```python
from build123d import *

# Parameters (mm, degrees)
SKETCH2_R               = 15
CUT_EXTRUDE1_DEPTH      = 10
CUT_EXTRUDE2_DEPTH      = 5.55
CUT_EXTRUDE2_DEPTH_BACK = 5.55


with BuildPart() as part:
    # Sketch1 → Revolve1 (revolve)
    with BuildSketch(Plane.XY, mode=Mode.PRIVATE) as revolve1_sk:
        Polygon((0, 0), (-50, 0), (-50, 30), (0, 15), align=None)
    revolve(revolve1_sk.sketch.rotate(Axis((0, 0, 0), (-1, 0, 0)), 90), axis=Axis((0, 0, 0), (-1, 0, 0)))

    # Sketch2 → Cut-Extrude1 (cut)
    with BuildSketch(Plane.ZY.offset(50)):
        Circle(SKETCH2_R)
    extrude(amount=-CUT_EXTRUDE1_DEPTH, mode=Mode.SUBTRACT)

    # Sketch4 → Cut-Extrude2 (cut, two sides: drawn at the far end of the back side and taken through both)
    with BuildSketch(Plane.XY.offset(-CUT_EXTRUDE2_DEPTH_BACK)):
        Polygon((0, 15), (0, 12), (-50, 27), (-50, 30), align=None)
        Polygon((0, -15), (0, -12), (-50, -27), (-50, -30), align=None)
    extrude(amount=CUT_EXTRUDE2_DEPTH + CUT_EXTRUDE2_DEPTH_BACK, mode=Mode.SUBTRACT)


solid = part.part
```
Could you check a few things on this model? Use its own coordinates, in mm. A direction names the side the tool comes from. Give positions to 0.01 mm unless a question says otherwise; leave off trailing zeros. Order: outer loops, then holes, each group sorted by start corner. A loop starts at its lowest first (then second) coordinate and runs counter-clockwise, first axis right, second up.
Q1. For faces 1 (the flat face through (-25, 21, 5.55)), 2 (the flat face through (-24.65, -19.395, -0.078)), 3 (the cylindrical face through (-45.07, 0.66, -14.985)), which set-ups out of +Z, -Z, +X, -X, +Y, -Y let a thin tool reach every point of the face, with its end or its side?
Q2. We'd pull the mould along Y, two halves only. Please class faces 4 (the flat face through (-25, 21, -5.55)), 5 (the flat face through (-40, 0, 0)), 6 (the conical face through (-24.65, -0.43, 22.39)): +Y half, -Y half, draft (parallel to the pull), parting line (faces both ways), or undercut.
Q3. Suppose I cut it at A-A, the plane y = 0. Write out the boundary of the cut face in (x, z).
Q4. Suppose I cut it at B-B, the plane z = 0. Write out the boundary of the cut face in (x, y).
Q5. I'm going to push flat-ended pins straight in: P1, Ø2, axis at x = -17.5, z = -6.5, coming from the +Y side; P2, Ø3, axis at x = -23, y = -20, coming from the +Z side; P3, Ø5, axis at x = -34.5, y = 23, coming from the -Z side; P4, Ø5, axis at x = -17, y = -22.5, coming from the +Z side. Where does each tip first touch, or does it pass through?
Q6. If I drill on line 1 along Z through (x, y) = (-47, 26.5); line 2 along X through (y, z) = (7, 0); line 3 along Y through (x, z) = (-46, 0), over which ranges is the centre line in solid material (lowest first)?
Solution:
1. face 1: +X, +Y
1. face 2: +X, -Y
1. face 3: -X
2. face 4: draft
2. face 5: undercut
2. face 6: parting line
3. outline: (-50, -30) - (0, -15) - (0, 15) - (-50, 30) - (-50, 15) - (-40, 15) - (-40, -15) - (-50, -15) - close
4. outline: (-50, -27) - (0, -12) - (0, 12) - (-50, 27) - (-50, 15) - (-40, 15) - (-40, -15) - (-50, -15) - close
5. P1: stops at y = 19.63
5. P2: stops at z = 11.86
5. P3: stops at z = -15.14
5. P4: passes through
6. line 1: z = -12.02 to -5.55, 5.55 to 12.02
6. line 2: x = -40 to 0
6. line 3: y = -25.8 to -15, 15 to 25.8
